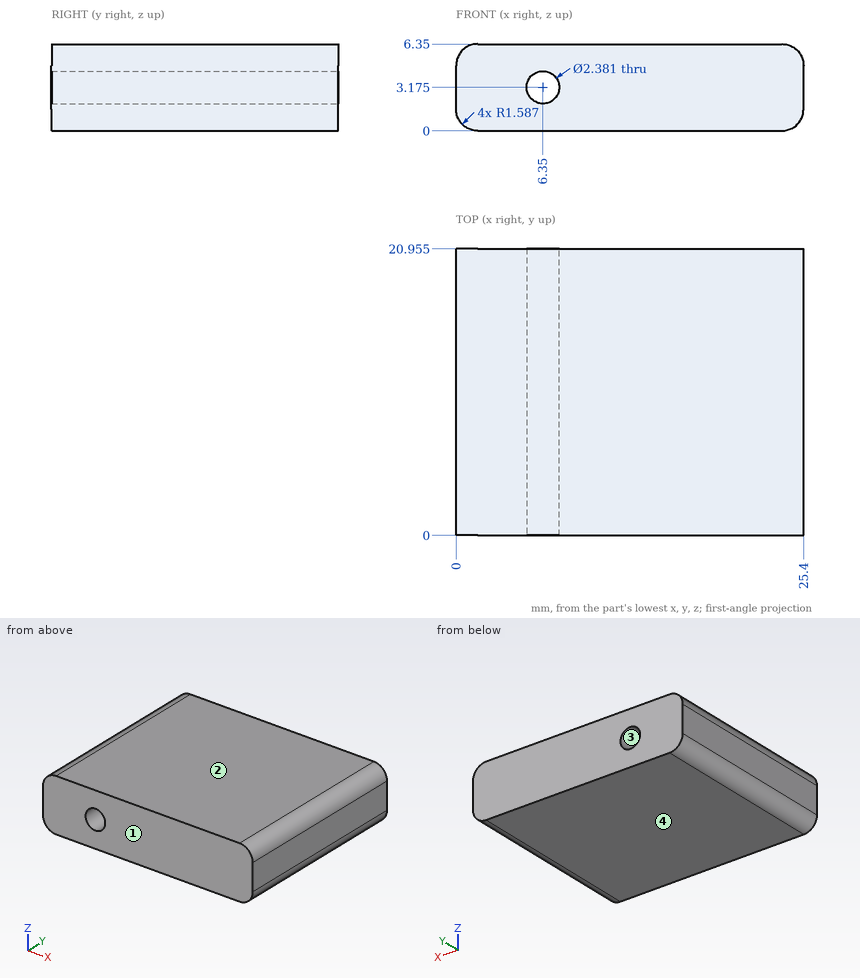
Design review of the part shown in the three views and the two pictorial views. Dimensions are in mm from the part's minimum x, y and z. Coordinates: 2 decimals unless noted, no trailing zeros.
(1) Wall thickness on probe 1 along X at (y, z) = (11.5, 1.5); probe 2 along X at (y, z) = (2.75, 3.5) (1 decimal); probe 3 along X at (y, z) = (12.75, 0.5): over which ranges is each line inside the solid? List them lowest first.
(2) For pin 1 Ø2.5 at (x, z) = (6.35, 3.175) entering from -Y, flat-tipped, find the tip position at first contact; note if it passes through.
(3) The part is to be moulded in two halves that separate along Z. For the marked faces 1, 2, 3 and 4, say which applies: +Z half, -Z half, draft (parallel to the pull), parting line (faces both ways), or undercut.
Answer sheet:
1. probe 1: x = 0 to 25.4
1. probe 2: x = 0 to 5.2, 7.5 to 25.4
1. probe 3: x = 0.43 to 24.97
2. pin 1: stops at y = 0
3. face 1: draft
3. face 2: +Z half
3. face 3: undercut
3. face 4: -Z half
